```python
from build123d import *

# Parameters (mm, degrees)
F1_DEPTH = 21.844
F2_SIZE  = 2.54
F3_R     = 5.08


with BuildPart() as f1:
    # F0 (on Top) → F1 (new body)
    with BuildSketch(Plane.XY):
        Polygon((26.936827, -12.972092), (26.936827, 12.972092), (6.652847, 29.148027), (-18.640863, 23.374903), (-29.897623, 0), (-18.640863, -23.374903), (6.652847, -29.148027), align=None)
    extrude(amount=F1_DEPTH)

    # F2
    f2_edges = [f1.edges().sort_by_distance(p)[0] for p in [
        (26.936827, 0, 21.844),
        (16.794837, -21.06006, 21.844),
        (-5.994008, -26.261465, 21.844),
        (-24.269243, -11.687451, 21.844),
        (-24.269243, 11.687451, 21.844),
        (-5.994008, 26.261465, 21.844),
        (16.794837, 21.06006, 21.844),
    ]]
    chamfer(f2_edges, length=F2_SIZE)

    # F3
    f3_edges = [f1.edges().sort_by_distance(p)[0] for p in [
        (16.794837, -21.06006, 0),
        (26.936827, 0, 0),
        (-5.994008, -26.261465, 0),
    ]]
    fillet(f3_edges, radius=F3_R)


solid = f1.part
```
Design review of the part built by this model. Coordinates are the model's own, in mm. Give positions to 0.01 mm unless a question says otherwise; leave off trailing zeros. Write each loop counter-clockwise with the first axis right and the second up, starting at its lowest first coordinate (ties: lowest second). Pieces come first, ordered by that corner, then holes. Notation, with made-up numbers: (55, 89) -> (79, 89) arc R16 cw to (79, 96) -> close; hole circle Ø5 at (25, 87.25). An arc over 180 degrees is marked (long way). Answer in a Markdown table with one row per item.
(1) To check wall thickness, follow probe 1 along X at (y, z) = (9, 19.5); probe 2 along X at (y, z) = (18, 13); probe 3 along Y at (x, z) = (-12, 18.75). State the ranges of each line that lie inside material, in increasing order.
Results:
| item | result |
|---|---|
| probe 1 | -25.35 to 26.74 |
| probe 2 | -21.23 to 20.63 |
| probe 3 | -24.89 to 24.89 |
(2) Consider section A-A (z = 9.75). State the section outline as (x, y) points, then the cut area to 3 significant figures.
Results:
| item | result |
|---|---|
| outline | (-29.9, 0) -> (-18.64, -23.37) -> (6.65, -29.15) -> (26.94, -12.97) -> (26.94, 12.97) -> (6.65, 29.15) -> (-18.64, 23.37) -> close |
| area | 2,450 mm2 |
(3) Mouldability with a two-part tool opening along Y and no side actions: class faces 1 (the flat face through (15.85, -20.17, 20.59)), 2 (the flat face through (-23.03, 11.292, 20.592)), 3 (the flat face through (25.65, -0.18, 20.59)) as +Y half, -Y half, draft (parallel to the pull), parting line (faces both ways), or undercut.
Results:
| item | result |
|---|---|
| face 1 | -Y half |
| face 2 | +Y half |
| face 3 | draft |
(4) Consider section B-B (y = -4.5). State the section outline as (x, z) points, then the cut area to 3 significant figures.
Results:
| item | result |
|---|---|
| outline | (-27.73, 0) -> (21.86, 0) arc R5.08 ccw to (26.94, 5.08) -> (26.94, 19.3) -> (24.4, 21.84) -> (-24.91, 21.84) -> (-27.73, 19.3) -> close |
| area | 1,180 mm2 |
(5) Clearance check with flat-ended pins moving along their axes: pin 1 (3 mm diameter, centred on x = 16.5, z = 10.5, fed in from -Y); pin 2 (8 mm diameter, centred on y = -2.5, z = 3.5, fed in from +X); pin 3 (10 mm diameter, centred on x = 1, z = 8.5, fed in from +Y); pin 4 (4 mm diameter, centred on x = -6.5, z = 15.5, fed in from -Y). State where each tip first meets the part, or that it passes through.
Results:
| item | result |
|---|---|
| pin 1 | y = -22.49 |
| pin 2 | x = 26.94 |
| pin 3 | y = 29 |
| pin 4 | y = -26.6 |
